The listing builds one solid part. Answer for the finished solid, in the listing's coordinates (mm). A direction names the side the tool comes from. Coordinates: 2 decimals unless noted, no trailing zeros. Loops run counter-clockwise (first coordinate to the right, second up) from the corner with the lowest first, then second, coordinate; pieces in that order, holes last. Notation, with made-up numbers: M 6,9 L 46,9 A20 cw 46,44 Z; hole C 23,-28.75 d3. An arc over 180 degrees is marked long. Return JSON: item names as keys, results as strings. Group by question number.
1. Section B-B (x = -15) is taken. Write down the section's boundary in (y, z), then the cut area to 3 significant figures.
2. Section D-D (y = 22.5) is taken. Count the separate pieces of the cut face and the enclosed holes in it, then the cut area to 3 significant figures.
3. Section C-C (z = -12.5) is taken. Write down the section's boundary in (x, y).
4. Which of the six approach directions +Z, -Z, +X, -X, +Y, -Y give full straight-line access (tool end or side, diameter ignored) to faces 1 (the face through (-31, 17, 9)), 2 (the face through (-42, 20, 21)), 3 (the face through (81.98, 23, 15))?
5. Straight lines are drawn through the part: L1, parallel to Z at x = -0.5, y = 19.5; L2, parallel to Y at x = -36, z = 28; L3, parallel to Y at x = -36, z = -12. For each, find the intervals that lie inside material, in ascending order. Write a range as from..to.
6. Section A-A (x = -36) is taken. Write down the section's boundary in (y, z), then the cut area to 3 significant figures.
7. Given P1, Ø12, axis at x = -36.5, y = 19.5, coming from the -Z side; P2, Ø19, axis at x = -36, y = 22.5, coming from the +Z side; P3, Ø18, axis at x = -29.5, z = -2, coming from the +Y side; P4, Ø18, axis at x = 26, z = -5.5, coming from the -Y side, each flat-ended and moving along its own axis, determine where each tip first touches the part or whether it passes through.
8. The mould has two halves that part along Z. Classify faces 4 (the face through (63.98, 23, 15)), 5 (the face through (14.99, 22.18, 0.52)), 6 (the face through (-13, 22, -30)): pulls with the +Z half, pulls with the -Z half, needs draft (parallel to the pull), parting line crosses it, or undercut.
```python
from build123d import *

# Parameters (mm, degrees)
BOSS_EXTRUDE1_DEPTH                                  = 45
CBORE_FOR_M24_HEX_SOCKET_HEAD_CAP_SCREW1_D           = 12
CBORE_FOR_M24_HEX_SOCKET_HEAD_CAP_SCREW1_DEPTH       = 21
CBORE_FOR_M24_HEX_SOCKET_HEAD_CAP_SCREW1_CBORE_D     = 24
CBORE_FOR_M24_HEX_SOCKET_HEAD_CAP_SCREW1_CBORE_DEPTH = 9
BOSS_EXTRUDE2_DEPTH                                  = 4.5
BOSS_EXTRUDE3_DEPTH                                  = 9
SKETCH7_W                                            = 60
SKETCH7_H                                            = 9
BOSS_EXTRUDE4_DEPTH                                  = 9
CUT_EXTRUDE2_START                                   = -60
CUT_EXTRUDE2_DEPTH                                   = 60
SKETCH9_R                                            = 7.5
CUT_EXTRUDE3_DEPTH                                   = 151.324191827
CUT_EXTRUDE4_DEPTH                                   = 149.198401551


# Read off the part's stored shape, not the designer's step: Cut-Extrude2
with BuildPart() as part:
    # Sketch1 → Boss-Extrude1 (new body)
    with BuildSketch(Plane(origin=(0, 0, 0), x_dir=(1, 0, 0), z_dir=(0, 1, 0))):
        with BuildLine():
            Line((0, -30), (-60, -30))
            Line((-60, -30), (-60, -9))
            Line((-60, -9), (-12, -9))
            ThreePointArc((-12, -9), (15, 0), (-12, 9))
            Line((-12, 9), (-60, 9))
            Line((-60, 9), (-60, 30))
            Line((-60, 30), (0, 30))
            ThreePointArc((0, 30), (30, 0), (0, -30))
        make_face()
    extrude(amount=BOSS_EXTRUDE1_DEPTH)

    # CBORE for M24 Hex Socket Head Cap Screw1
    with Locations(Plane.XY.offset(30)):
        with Locations((-36, 22.5)):
            cbore_for_m24_hex_socket_head_cap_screw1 = CounterBoreHole(CBORE_FOR_M24_HEX_SOCKET_HEAD_CAP_SCREW1_D / 2, CBORE_FOR_M24_HEX_SOCKET_HEAD_CAP_SCREW1_CBORE_D / 2, CBORE_FOR_M24_HEX_SOCKET_HEAD_CAP_SCREW1_CBORE_DEPTH, depth=CBORE_FOR_M24_HEX_SOCKET_HEAD_CAP_SCREW1_DEPTH)

    # Mirror1: CBORE for M24 Hex Socket Head Cap Screw1 across plane
    add(cbore_for_m24_hex_socket_head_cap_screw1.mirror(Plane.XY), mode=Mode.SUBTRACT)

    # Sketch4 → Boss-Extrude2 (add, symmetric)
    with BuildSketch(Plane(origin=(0, 22.5, 0), x_dir=(1, 0, 0), z_dir=(0, 1, 0))):
        with BuildLine():
            Line((0, 30), (90, 30))
            Line((90, 30), (90, -30))
            Line((90, -30), (0, -30))
            ThreePointArc((0, -30), (30, 0), (0, 30))
        make_face()
    extrude(amount=BOSS_EXTRUDE2_DEPTH, both=True)



with BuildPart() as body_2:
    # Sketch6 → Boss-Extrude3 (new body)
    with BuildSketch(Plane(origin=(31.5, -31.5, 0), x_dir=(0.7071067811865462, 0.7071067811865489, 0), z_dir=(0.7071067811865489, -0.7071067811865462, 0))):
        with BuildLine():
            Line((82.731493399, 30), (82.731493399, -30))
            Line((82.731493399, -30), (132.264035588, -14.298813283))
            ThreePointArc((132.264035588, -14.298813283), (142.731493399, 0), (132.264035588, 14.298813283))
            Line((132.264035588, 14.298813283), (82.731493399, 30))
        make_face()
    extrude(amount=BOSS_EXTRUDE3_DEPTH)


with BuildPart() as part_1:
    add(part.part)

    add(body_2.part)  # Boss-Extrude4 merges body 2
    # Sketch7 → Boss-Extrude4 (add)
    with BuildSketch(Plane(origin=(58.5, 58.5, 0), x_dir=(0, 0, 1), z_dir=(-0.7071067811865462, -0.7071067811865488, 0))):
        with Locations((0, -49.047727215)):
            Rectangle(SKETCH7_W, SKETCH7_H)
    extrude(amount=BOSS_EXTRUDE4_DEPTH)

    # Cut-Extrude2 outline → Cut-Extrude2 (cut)
    with BuildSketch(Plane.XY.offset(30).offset(CUT_EXTRUDE2_START)):
        Polygon((90, 14.272077939), (93.727922061, 18), (86.272077939, 18), align=None)
    extrude(amount=CUT_EXTRUDE2_DEPTH, mode=Mode.SUBTRACT)

    # Sketch9 → Cut-Extrude3 (cut, through all)
    with BuildSketch(Plane(origin=(31.5, -31.5, 0), x_dir=(0, 0, 1), z_dir=(-0.7071067811865488, 0.7071067811865464, 0))):
        with Locations(Location((0, 127.731493399, 0), (0, 0, 270))):
            Circle(SKETCH9_R)
    extrude(amount=-CUT_EXTRUDE3_DEPTH, mode=Mode.SUBTRACT)

    # Sketch10 → Cut-Extrude4 (cut, through all)
    with BuildSketch(Plane(origin=(0, 27, 0), x_dir=(1, 0, 0), z_dir=(0, 1, 0))):
        with BuildLine():
            ThreePointArc((81.979848708, 0), (72.979848708, 9), (63.979848708, 0))
            Line((63.979848708, 0), (63.979848708, -30))
            Line((63.979848708, -30), (81.979848708, -30))
            Line((81.979848708, -30), (81.979848708, 0))
        make_face()
    extrude(amount=-CUT_EXTRUDE4_DEPTH, mode=Mode.SUBTRACT)


solid = part_1.part
```
Worked out:
{
 "1": {"outline": "M 0,-30 L 45,-30 L 45,-9 L 0,-9 Z; M 0,9 L 45,9 L 45,30 L 0,30 Z", "area": "1,890 mm^2"},
 "2": {"separate pieces": "3", "enclosed holes": "0", "area": "6,570 mm^2"},
 "3": {"outline": "M -60,0 L -8.29,0 L -8.29,45 L -60,45 Z; M 8.29,0 L 27.27,0 L 27.27,18 L 93.73,18 L 134.05,58.32 L 127.68,64.68 L 90,27 L 27.27,27 L 27.27,45 L 8.29,45 Z; hole C -36,22.5 d12"},
 "4": {"face 1": "-X, +Y, -Y", "face 2": "+Z", "face 3": "+Z, +Y, -Y"},
 "5": {"L1": "-30..-14.99, 14.99..30", "L2": "0..10.5, 34.5..45", "L3": "0..16.5, 28.5..45"},
 "6": {"outline": "M 0,-30 L 10.5,-30 L 10.5,-21 L 16.5,-21 L 16.5,-9 L 0,-9 Z; M 0,9 L 16.5,9 L 16.5,21 L 10.5,21 L 10.5,30 L 0,30 Z; M 28.5,-21 L 34.5,-21 L 34.5,-30 L 45,-30 L 45,-9 L 28.5,-9 Z; M 28.5,9 L 45,9 L 45,30 L 34.5,30 L 34.5,21 L 28.5,21 Z", "area": "1,170 mm^2"},
 "7": {"P1": "z = -21", "P2": "z = 21", "P3": "y = 45", "P4": "y = 0"},
 "8": {"face 4": "needs draft", "face 5": "undercut", "face 6": "pulls with the -Z half"}
}
